The figure shows three views and two pictorial views of one solid part (mm, origin at its lowest corner). Answer the questions. A direction names the side the tool comes from. Round coordinates to 2 decimals unless told otherwise and drop trailing zeros. Loops run counter-clockwise (first coordinate to the right, second up) from the corner with the lowest first, then second, coordinate; pieces in that order, holes last. Notation, with made-up numbers: (17.5, -15.5) -> (32.5, -15.5) arc R35 cw to (32.5, 19.5) -> close; hole circle Ø4 at (7.5, 29). An arc over 180 degrees is marked (long way). Put each result on its own line as item: value.
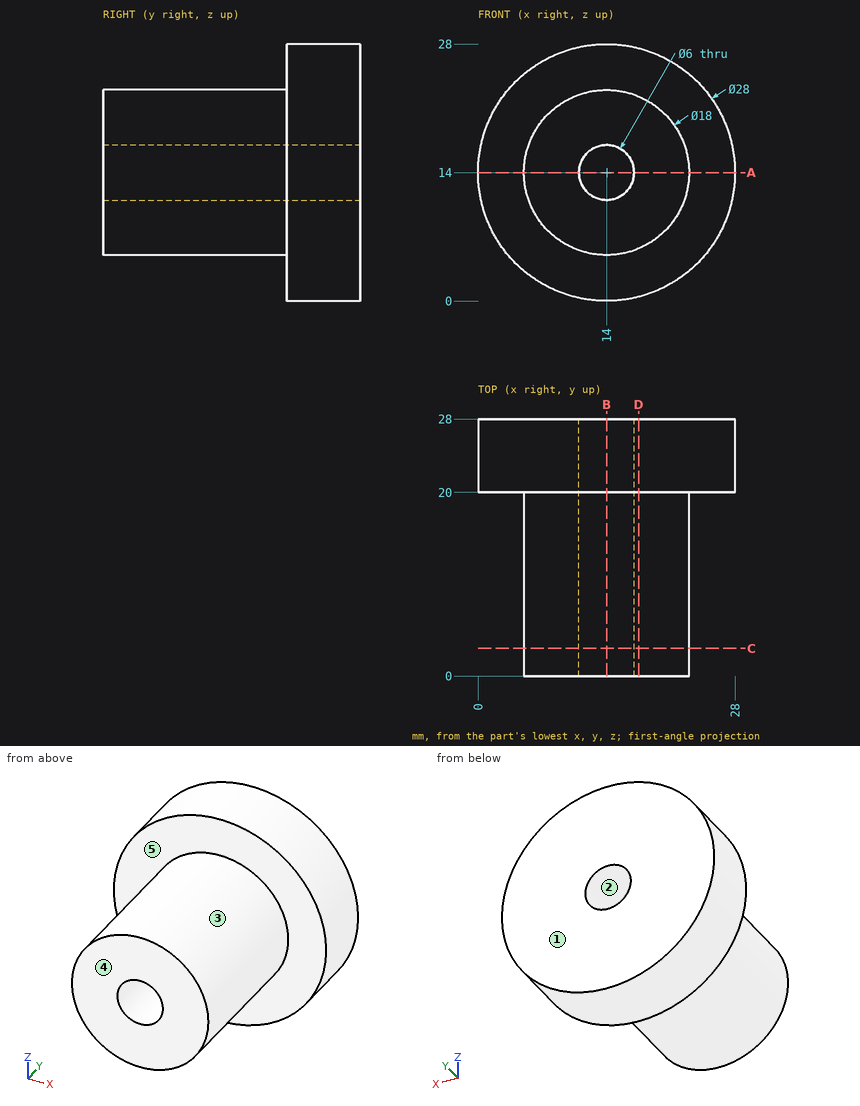
Item 1: For a pull along X with two mould halves and no side action, classify the marked faces 1, 2 and 3 as pulls with the +X half, pulls with the -X half, needs draft (parallel to the pull), parting line crosses it, or undercut.
Derived:
face 1: needs draft
face 2: undercut
face 3: parting line crosses it
Item 2: Find the intervals of material crossed by line 1 along Z through (x, y) = (14, 21.5); line 2 along Z through (x, y) = (14, 9); line 3 along Y through (x, z) = (6.75, 23), in increasing order.
Derived:
line 1: z = 0 to 11, 17 to 28
line 2: z = 5 to 11, 17 to 23
line 3: y = 20 to 28
Item 3: The part is cut by section C-C (y = 3). Determine the outline of the cut face in (x, z).
Derived:
outline: circle Ø18 at (14, 14); hole circle Ø6 at (14, 14)
Item 4: Which of the six approach directions +Z, -Z, +X, -X, +Y, -Y give full straight-line access (tool end or side, diameter ignored) to the marked faces 4 and 5?
Derived:
face 4: +Z, -Z, +X, -X, -Y
face 5: -Y
Item 5: Flat-ended cylindrical pins translate along their axes: pin 1 Ø1 at (x, y) = (17.5, 3) entering from +Z; pin 2 Ø10 at (x, y) = (24.5, 21) entering from +Z; pin 3 Ø6 at (x, y) = (7.5, 6.5) entering from +Z. Find the tip coordinate at first contact, or state that the pin passes through.
Derived:
pin 1: stops at z = 22.49
pin 2: stops at z = 26.87
pin 3: stops at z = 22.29
Item 6: The part is cut by section A-A (z = 14). Determine the outline of the cut face in (x, y).
Derived:
outline: (0, 20) -> (5, 20) -> (5, 0) -> (11, 0) -> (11, 28) -> (0, 28) -> close; (17, 0) -> (23, 0) -> (23, 20) -> (28, 20) -> (28, 28) -> (17, 28) -> close
Item 7: The part is cut by section B-B (x = 14). Determine the outline of the cut face in (y, z).
Derived:
outline: (0, 5) -> (20, 5) -> (20, 0) -> (28, 0) -> (28, 11) -> (0, 11) -> close; (0, 17) -> (28, 17) -> (28, 28) -> (20, 28) -> (20, 23) -> (0, 23) -> close
Item 8: The part is cut by section D-D (x = 17.5). Determine the outline of the cut face in (y, z), then the cut area to 3 significant figures.
Derived:
outline: (0, 5.71) -> (20, 5.71) -> (20, 0.44) -> (28, 0.44) -> (28, 27.56) -> (20, 27.56) -> (20, 22.29) -> (0, 22.29) -> close
area: 549 mm^2
